```python
from build123d import *

# Parameters (mm, degrees)
RESSALTO_EXTRUS_O1_DEPTH = 171.8
ESBO_O2_R                = 1.75
ESBO_O2_R_2              = 4.5
ESBO_O2_R_3              = 2.5
ESBO_O2_R_4              = 1.5
ESBO_O2_W                = 48.2
ESBO_O2_H                = 82
CORTE_EXTRUS_O1_DEPTH    = 91.8
ESBO_O3_R                = 1.5
CORTE_EXTRUS_O2_DEPTH    = 91.8


with BuildPart() as part:
    # Esboço1 → Ressalto-extrusão1 (new body)
    with BuildSketch(Plane.XY):
        Polygon((0, 0), (36, 0), (95.500769823, -39.667179882), (93.03235395, -43.369803692), (36.677648412, -5.8), (0, -5.8), align=None)
    extrude(amount=RESSALTO_EXTRUS_O1_DEPTH)

    # Esboço2 → Corte-extrusão1 (cut)
    with BuildSketch(Plane(origin=(11.076923077, 16.615384615, 0), x_dir=(0.8320502943378437, -0.5547001962252291, 0), z_dir=(0.5547001962252291, 0.8320502943378437, 0))):
        with Locations(Location((44.779323351, -112.8, 0), (0, 0, 180))):
            Circle(ESBO_O2_R)
        with Locations(Location((86.639323351, -112.8, 0), (0, 0, 180))):
            Circle(ESBO_O2_R)
        with Locations(Location((44.779323351, -23.2, 0), (0, 0, 180))):
            Circle(ESBO_O2_R)
        with Locations(Location((86.639323351, -23.2, 0), (0, 0, 180))):
            Circle(ESBO_O2_R)
        with Locations(Location((77.664836105, -137, 0), (0, 0, 180))):
            Circle(ESBO_O2_R_2)
        with Locations(Location((47.118170034, -137, 0), (0, 0, 180))):
            Circle(ESBO_O2_R_2)
        with Locations(Location((62.164836105, -159.5, 0), (0, 0, 180))):
            Circle(ESBO_O2_R_3)
        with Locations(Location((96.064836105, -164.4, 0), (0, 0, 180))):
            Circle(ESBO_O2_R_4)
        with Locations(Location((96.064836105, -7.4, 0), (0, 0, 180))):
            Circle(ESBO_O2_R_4)
        with Locations((65.983311741, -68)):
            Rectangle(ESBO_O2_W, ESBO_O2_H)
    extrude(amount=-CORTE_EXTRUS_O1_DEPTH, mode=Mode.SUBTRACT)

    # Esboço3 → Corte-extrusão2 (cut)
    with BuildSketch(Plane(origin=(0, 0, 0), x_dir=(1, 0, 0), z_dir=(0, 1, 0))):
        with Locations(Location((5, -166.9, 0), (0, 0, 270))):
            Circle(ESBO_O3_R)
        with Locations(Location((5, -4.9, 0), (0, 0, 270))):
            Circle(ESBO_O3_R)
    extrude(amount=-CORTE_EXTRUS_O2_DEPTH, mode=Mode.SUBTRACT)


solid = part.part
```
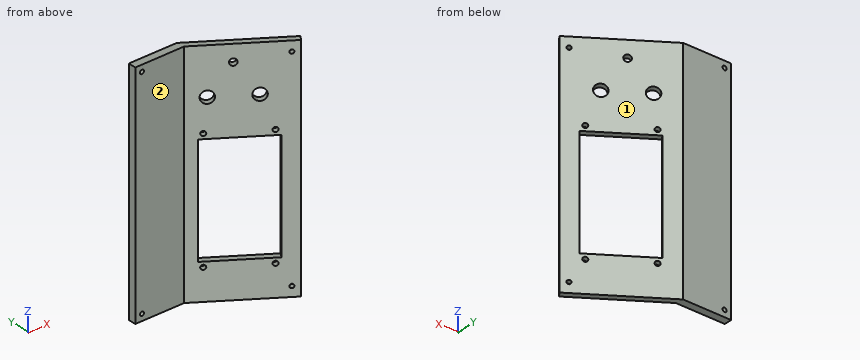
Read the model definition and answer for the solid it produces. Units are mm, in the model's axes. Face numbers are marked on the shaded views. A direction names the side the tool comes from. Coordinates: 2 decimals unless noted, no trailing zeros. Write each loop counter-clockwise with the first axis right and the second up, starting at its lowest first coordinate (ties: lowest second). Pieces come first, ordered by that corner, then holes. Notation, with made-up numbers: (32.25, 12) - (59.25, 12) arc R26 ccw to (59.25, 38) - close; hole circle Ø1 at (25.25, -3). An arc over 180 degrees is marked (long way). Answer as a JSON object with one key per item and string values. Group by question number.
1. A cutting plane is placed at A-A (z = 96). Determine the outline of the cut face in (x, y).
2. Which of the six approach directions +Z, -Z, +X, -X, +Y, -Y give full straight-line access (tool end or side, diameter ignored) to the marked faces 1 and 2?
3. A cutting plane is placed at B-B (y = -4). Determine the outline of the cut face in (x, z), plus the area to 3 significant figures.
4. Consider L1, parallel to Z at x = 73, y = -25; L2, parallel to X at y = -3, z = 166.9; L3, parallel to Y at x = 31, z = 119.5. Determine where each line is inside the solid, lowest interval first. Write a range as [from, to].
5. A cutting plane is placed at D-D (z = 122.5). Determine the outline of the cut face in (x, y).
6. A cutting plane is placed at C-C (x = 29.5). Determine the outline of the cut face in (y, z), plus the area to 3 significant figures.
7. Each of these flat-tipped pins is pushed along its axis until it touches: P1, Ø2.5, axis at x = 5, z = 4.9, coming from the -Y side; P2, Ø11, axis at x = 12, z = 68, coming from the -Y side; P3, Ø12, axis at y = -15.5, z = 148, coming from the -X side; P4, Ø4, axis at y = -6, z = 138.5, coming from the +X side. Where does it stop, or does it pass through?
Worked out:
{
 "1": {"outline": "(0, -5.8) - (36.68, -5.8) - (43.46, -10.32) - (45.93, -6.62) - (36, 0) - (0, 0) - close; (83.56, -37.06) - (93.03, -43.37) - (95.5, -39.67) - (86.03, -33.35) - close"},
 "2": {"face 1": "+Z, -Z, +X, +Y", "face 2": "+Z, -Z, -X, -Y"},
 "3": {"outline": "(0, 0) - (42, 0) - (42, 171.8) - (0, 171.8) - close; hole circle Ø3 at (5, 4.9); hole circle Ø3 at (5, 166.9)", "area": "7,200 mm²"},
 "4": {"L1": "z = [0, 27], [109, 133.7], [140.3, 171.8]", "L2": "x = [0, 3.5], [6.5, 40.5]", "L3": "y = [-5.8, 0]"},
 "5": {"outline": "(0, -5.8) - (36.68, -5.8) - (93.03, -43.37) - (95.5, -39.67) - (36, 0) - (0, 0) - close"},
 "6": {"outline": "(-5.8, 0) - (0, 0) - (0, 171.8) - (-5.8, 171.8) - close", "area": "996 mm²"},
 "7": {"P1": "passes through", "P2": "stops at y = -5.8", "P3": "stops at x = 42.23", "P4": "stops at x = 47.33"}
}
